The model under review builds one solid part; all positions refer to its coordinate system, in mm. Face numbers are marked on the shaded views. A direction names the side the tool comes from. Give positions to 0.01 mm unless a question says otherwise; leave off trailing zeros. Loops run counter-clockwise (first coordinate to the right, second up) from the corner with the lowest first, then second, coordinate; pieces in that order, holes last. Notation, with made-up numbers: M 36.25,45 L 72.25,45 A30 cw 72.25,76 Z; hole C 2.25,26.25 d1. An arc over 180 degrees is marked long. Put each result on its own line as item: value. Start each with the question number.
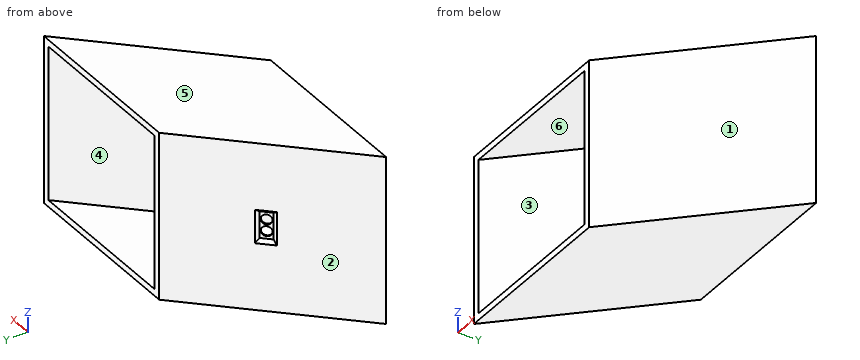
from build123d import *

# Parameters (mm, degrees)
SALIENTE_EXTRUIR1_DEPTH = 2
SALIENTE_EXTRUIR2_DEPTH = 46
SALIENTE_EXTRUIR3_DEPTH = 2
CROQUIS5_R              = 1.5
CORTAR_EXTRUIR1_DEPTH   = 1.414213562
CROQUIS8_W              = 10
CROQUIS8_H              = 5.5
CORTAR_EXTRUIR2_DEPTH   = 1
CORTAR_EXTRUIR2_DRAFT   = -45


with BuildPart() as part:
    # Croquis2 → Saliente-Extruir1 (new body)
    with BuildSketch(Plane.XY):
        Polygon((-42.342007435, -30.353159851), (7.657992565, -30.353159851), (-32.342007435, -70.353159851), (-82.342007435, -70.353159851), align=None)
    extrude(amount=SALIENTE_EXTRUIR1_DEPTH)

    # Croquis3 → Saliente-Extruir2 (add)
    with BuildSketch(Plane(origin=(0, 0, 0), x_dir=(-1, 0, 0), z_dir=(0, 0, -1))):
        Polygon((-5.657992565, -30.353159851), (-7.657992565, -30.353159851), (32.342007435, -70.353159851), (34.342007435, -70.353159851), align=None)
        Polygon((42.342007435, -30.353159851), (40.342007435, -30.353159851), (80.342007435, -70.353159851), (82.342007435, -70.353159851), align=None)
    extrude(amount=SALIENTE_EXTRUIR2_DEPTH)

    # Croquis4 → Saliente-Extruir3 (add)
    with BuildSketch(Plane(origin=(0, 0, -46), x_dir=(-1, 0, 0), z_dir=(0, 0, -1))):
        Polygon((-7.657992565, -30.353159851), (42.342007435, -30.353159851), (82.342007435, -70.353159851), (32.342007435, -70.353159851), align=None)
    extrude(amount=SALIENTE_EXTRUIR3_DEPTH)

    # Croquis5 → Cortar-Extruir1 (cut)
    with BuildSketch(Plane(origin=(-5.994423792, 5.994423792, 0), x_dir=(0, 0, 1), z_dir=(-0.7071067811865438, 0.7071067811865513, 0))):
        with Locations(Location((-24.75, -77.971788243, 0), (0, 0, 270))):
            Circle(CROQUIS5_R)
        with Locations(Location((-21.25, -77.971788243, 0), (0, 0, 270))):
            Circle(CROQUIS5_R)
    extrude(amount=-CORTAR_EXTRUIR1_DEPTH, mode=Mode.SUBTRACT)


with BuildPart() as cortar_extruir2_tool:
    # Croquis8 → Cortar-Extruir2 (with draft: the straight prism first)
    with BuildSketch(Plane(origin=(-5.994423792, 5.994423792, 0), x_dir=(0, 0, 1), z_dir=(-0.7071067811865438, 0.7071067811865513, 0))):
        with Locations((-23, -77.971788243)):
            Rectangle(CROQUIS8_W, CROQUIS8_H)
    extrude(amount=-CORTAR_EXTRUIR2_DEPTH)
    # Cortar-Extruir2: the draft: its side faces are tilted about the plane it starts from
    cortar_extruir2_sides = [cortar_extruir2_tool.faces().sort_by_distance(p)[0] for p in [
        (-62.719794257, -51.438053455, -23),
        (-60.775250609, -49.493509806, -18),
        (-58.83070696, -47.548966158, -23),
        (-60.775250609, -49.493509806, -28),
    ]]
    draft(cortar_extruir2_sides, Plane(origin=(-5.994423792, 5.994423792, 0), x_dir=(0, 0, 1), z_dir=(-0.7071067811865438, 0.7071067811865513, 0)), CORTAR_EXTRUIR2_DRAFT)


with BuildPart() as part_1:
    add(part.part)

    # Cortar-Extruir2: cut by cortar_extruir2_tool
    add(cortar_extruir2_tool.part, mode=Mode.SUBTRACT)


solid = part_1.part
(1) For the marked faces 4, 5 and 6, list the 3-axis set-ups (+Z, -Z, +X, -X, +Y, -Y) from which the entire face can be reached by the end or side of a thin tool; tool diameter is ignored.
(2) We need section B-B, the plane z = -38. Write out the cut boundary in (x, y), plus the area to 3 significant figures.
(3) We need section D-D, the plane x = -28.5. Write out the cut boundary in (y, z).
(4) We need section C-C, the plane y = -33. Write out the cut boundary in (x, z), plus the area to 3 significant figures.
(5) To check wall thickness, follow L1, parallel to Z at x = -45.5, y = -61; L2, parallel to X at y = -36, z = -10; L3, parallel to X at y = -51.5, z = -30.5. State the ranges of each line that lie inside material, in increasing order. Write a range as [from, to].
(6) Draft analysis for pull direction X (two halves, no side actions). For the marked faces 1, 2 and 3, state which applies: +X half, -X half, draft (parallel to the pull), parting line (faces both ways), or undercut.
(7) We need section A-A, the plane x = -37.5. Write out the cut boundary in (y, z), plus the area to 3 significant figures.
(8) Insertion check: pin 1 (4 mm diameter, centred on x = -45, z = -9.5, fed in from -Y); pin 2 (3 mm diameter, centred on y = -38, z = -29.5, fed in from +X); pin 3 (5 mm diameter, centred on y = -65, z = -36, fed in from -X); pin 4 (1.5 mm diameter, centred on x = -36, z = -13, fed in from -Y). Each pin has a flat end and moves straight along its axis. Give the tip position at first contact, or say it passes through.
Check sheet entries:
1. face 4: +Y
1. face 5: +Z, +X, -X, +Y, -Y
1. face 6: none
2. outline: M -82.34,-70.35 L -80.34,-70.35 L -40.34,-30.35 L -42.34,-30.35 Z; M -34.34,-70.35 L -32.34,-70.35 L 7.66,-30.35 L 5.66,-30.35 Z
2. area: 160 mm²
3. outline: M -66.51,-48 L -30.35,-48 L -30.35,-46 L -64.51,-46 L -64.51,0 L -30.35,0 L -30.35,2 L -66.51,2 Z
4. outline: M -44.99,-48 L 5.01,-48 L 5.01,2 L -44.99,2 Z; hole M -42.99,-46 L 3.01,-46 L 3.01,0 L -42.99,0 Z
4. area: 384 mm²
5. L1: z = [-48, -46], [0, 2]
5. L2: x = [-47.99, -45.99], [0.01, 2.01]
5. L3: x = [-63.49, -61.49], [-15.49, -13.49]
6. face 1: +X half
6. face 2: -X half
6. face 3: undercut
7. outline: M -70.35,-48 L -30.35,-48 L -30.35,-46 L -70.35,-46 Z; M -70.35,0 L -30.35,0 L -30.35,2 L -70.35,2 Z
7. area: 160 mm²
8. pin 1: stops at y = -37.01
8. pin 2: stops at x = 1.51
8. pin 3: stops at x = -79.49
8. pin 4: passes through
